from build123d import *

# Parameters (mm, degrees)
SKETCH1_R               = 15
BOSS_EXTRUDE1_DEPTH     = 28
SKETCH2_R               = 10
CUT_EXTRUDE1_DEPTH      = 27
SKETCH3_R               = 11
CUT_EXTRUDE2_DEPTH      = 12
CUT_EXTRUDE3_DEPTH      = 36.128336141
CUT_EXTRUDE3_DEPTH_BACK = 36.128336141
SKETCH4_R               = 2.5
CHAMFER1_SIZE           = 0.5


with BuildPart() as part:
    # Sketch1 → Boss-Extrude1 (new body)
    with BuildSketch(Plane(origin=(0, 0, 0), x_dir=(1, 0, 0), z_dir=(0, 1, 0))):
        with Locations(Location((0, 0, 0), (0, 0, 270))):
            Circle(SKETCH1_R)
    extrude(amount=BOSS_EXTRUDE1_DEPTH)

    # Sketch2 → Cut-Extrude1 (cut)
    with BuildSketch(Plane(origin=(0, 28, 0), x_dir=(1, 0, 0), z_dir=(0, 1, 0))):
        with Locations(Location((0, 0, 0), (0, 0, 270))):
            Circle(SKETCH2_R)
    extrude(amount=-CUT_EXTRUDE1_DEPTH, mode=Mode.SUBTRACT)

    # Sketch3 → Cut-Extrude2 (cut)
    with BuildSketch(Plane(origin=(0, 28, 0), x_dir=(1, 0, 0), z_dir=(0, 1, 0))):
        with Locations(Location((0, 0, 0), (0, 0, 270))):
            Circle(SKETCH3_R)
    extrude(amount=-CUT_EXTRUDE2_DEPTH, mode=Mode.SUBTRACT)

    # Sketch4 → Cut-Extrude3 (cut, two sides: drawn at the far end of the back side and taken through both)
    with BuildSketch(Plane(origin=(0, 0, 0), x_dir=(0, 0, -1), z_dir=(1, 0, 0)).offset(-CUT_EXTRUDE3_DEPTH_BACK)):
        with Locations((0, 12)):
            Circle(SKETCH4_R)
    extrude(amount=CUT_EXTRUDE3_DEPTH + CUT_EXTRUDE3_DEPTH_BACK, mode=Mode.SUBTRACT)

    # Chamfer1
    chamfer1_edges = [part.edges().sort_by_distance(p)[0] for p in [
        (0, 28, -11),
        (0, 28, -15),
    ]]
    chamfer(chamfer1_edges, length=CHAMFER1_SIZE)


solid = part.part
The listing builds one solid part. Answer for the finished solid, in the listing's coordinates (mm). A direction names the side the tool comes from. Coordinates: 2 decimals unless noted, no trailing zeros. Write each loop counter-clockwise with the first axis right and the second up, starting at its lowest first coordinate (ties: lowest second). Pieces come first, ordered by that corner, then holes. Notation, with made-up numbers: (-14, 68) - (44, 68) arc R21 ccw to (44, 106) - close; hole circle Ø5 at (74.25, 78). An arc over 180 degrees is marked (long way). Return JSON: item names as keys, results as strings.
1. Each of these flat-tipped pins is pushed along its axis until it touches: pin 1 Ø3 at (x, y) = (-10, 23) entering from +Z; pin 2 Ø2 at (y, z) = (7, 10) entering from +X; pin 3 Ø6 at (x, y) = (-5.5, 11) entering from -Z. Where does it stop, or does it pass through?
Final values:
{"pin 1": "z = 12.36", "pin 2": "x = 12", "pin 3": "z = -14.79"}
2. The part is cut by section C-C on y = 5.75. Determine the outline of the cut face in (x, z).
Final values:
{"outline": "circle Ø30 at (0, 0); hole circle Ø20 at (0, 0)"}
3. The part is cut by section B-B on x = 0. Determine the outline of the cut face in (y, z), then the cut area to 4 significant figures.
Final values:
{"outline": "(0, -15) - (27.5, -15) - (28, -14.5) - (28, -11.5) - (27.5, -11) - (16, -11) - (16, -10) - (1, -10) - (1, 10) - (16, 10) - (16, 11) - (27.5, 11) - (28, 11.5) - (28, 14.5) - (27.5, 15) - (0, 15) - close", "area": "275.5 mm^2"}
4. For a pull along Z with two mould halves and no side action, classify faces 1 (the face through (0, 0, 0)), 2 (the face through (12.3, 14.48, 0.33)), 3 (the face through (-14.643, 13.558, -3.252)) as +Z half, -Z half, draft (parallel to the pull), parting line (faces both ways), or undercut.
Final values:
{"face 1": "draft", "face 2": "undercut", "face 3": "parting line"}
5. Which of the six approach directions +Z, -Z, +X, -X, +Y, -Y give full straight-line access (tool end or side, diameter ignored) to faces 4 (the face through (-10, 16, 2)), 5 (the face through (-12.38, 9.56, 0.54))?
Final values:
{"face 4": "+Y", "face 5": "+X, -X"}
6. Consider line 1 along X through (y, z) = (19.75, 0); line 2 along Z through (x, y) = (-5.5, 3.5); line 3 along X through (y, z) = (14.75, -2.5). Determine where each line is inside the solid, lowest interval first.
Final values:
{"line 1": "-15 to -11, 11 to 15", "line 2": "-13.96 to -8.35, 8.35 to 13.96", "line 3": "-14.79 to -9.68, 9.68 to 14.79"}
7. The part is cut by section A-A on z = 0. Determine the outline of the cut face in (x, y).
Final values:
{"outline": "(-15, 0) - (15, 0) - (15, 9.5) - (10, 9.5) - (10, 1) - (-10, 1) - (-10, 9.5) - (-15, 9.5) - close; (-15, 14.5) - (-10, 14.5) - (-10, 16) - (-11, 16) - (-11, 27.5) - (-11.5, 28) - (-14.5, 28) - (-15, 27.5) - close; (10, 14.5) - (15, 14.5) - (15, 27.5) - (14.5, 28) - (11.5, 28) - (11, 27.5) - (11, 16) - (10, 16) - close"}
8. The part is cut by section D-D on y = 12. Determine the outline of the cut face in (x, z), then the cut area to 3 significant figures.
Final values:
{"outline": "(-14.79, -2.5) arc R15 ccw to (14.79, -2.5) - (9.68, -2.5) arc R10 cw to (-9.68, -2.5) - close; (-14.79, 2.5) - (-9.68, 2.5) arc R10 cw to (9.68, 2.5) - (14.79, 2.5) arc R15 ccw to start", "area": "342 mm^2"}
